Geometry: final body of the model. Coordinates: model frame, mm. Give positions to 0.01 mm unless a question says otherwise; leave off trailing zeros. Write each loop counter-clockwise with the first axis right and the second up, starting at its lowest first coordinate (ties: lowest second). Pieces come first, ordered by that corner, then holes.
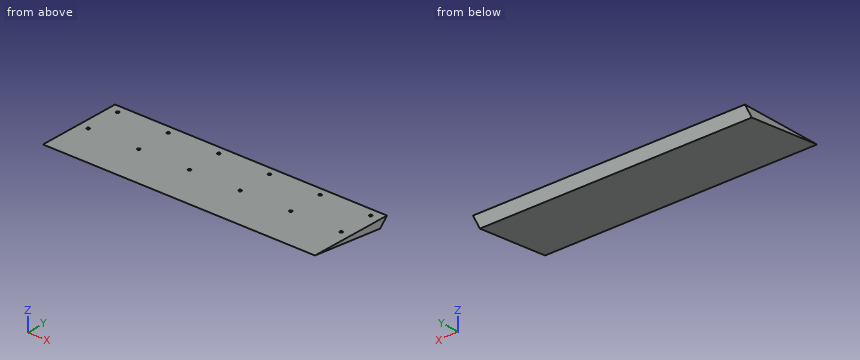
Autodesk Fusion 360 part; units mm, degrees
sketch "Sketch1" plane through (0, 0, 0) normal (0, 0, 1) x (1, 0, 0)
  line L0 (-217, 72) -> (217, 72)
  line L1 (217, 72) -> (217, -62)
  line L2 (217, -62) -> (-217, -62)
  line L3 (-217, -62) -> (-217, 72)
extrude "Extrude4" add sketch "Sketch1" against normal blind 230
sketch "Sketch4" plane through (-217, 0, 0) normal (-1, 0, 0) x (0, -1, 0)
  line L0 (62, 0) -> (-72, 0)
  line L1 (-72, 0) -> (-72, -230)
  line L2 (-72, -230) -> (62, -230)
  line L3 (62, -230) -> (62, 0)
  line L4 (62, 0) -> (-29, 0) construction
  line L5 (-72, 0) -> (-59.2555, -12.7445)
  line L6 (-72, 0) -> (-53.9766, 0) construction
  line L7 (62, 0) -> (-59.2555, -12.7445)
  line L8 (62, 0) -> (-59.9234, 0) construction
  dimension "d30" = 45
  dimension "d31" = 6
extrude "Extrude5" cut sketch "Sketch4" against normal blind 520 contours L1 L2 L3 L5 L7
sketch "Sketch5" plane through (0, 0, 0) normal (0, 0, 1) x (-1, 0, 0)
  line L0 (217, 62) -> (-217, 62)
  line L1 (-217, 62) -> (-217, -72)
  line L2 (-217, -72) -> (217, -72)
  line L3 (217, -72) -> (217, 62)
  circle A0 centre (202, -59.25) radius 2.25
  circle A1 centre (121.2, -59.25) radius 2.25
  circle A2 centre (40.4, -59.25) radius 2.25
  circle A3 centre (-40.4, -59.25) radius 2.25
  circle A4 centre (-121.2, -59.25) radius 2.25
  circle A5 centre (-202, -59.25) radius 2.25
  circle A6 centre (202, -4.5) radius 2.25
  circle A7 centre (121.2, -4.5) radius 2.25
  circle A8 centre (40.4, -4.5) radius 2.25
  circle A9 centre (-40.4, -4.5) radius 2.25
  circle A10 centre (-121.2, -4.5) radius 2.25
  circle A11 centre (-202, -4.5) radius 2.25
  dimension "d34" = 4.5
  dimension "d35" = 12.75
  dimension "d36" = 15
  dimension "d39" = -404
  dimension "d40" = 0
  dimension "d41" = 4.5
  dimension "d42" = 66.5
  dimension "d43" = 15
  dimension "d46" = -404
  dimension "d47" = 0
extrude "Extrude6" cut sketch "Sketch5" against normal blind 6 contours A0 | A1 | A2 | A3 | A4 | A5 | A6 | A7 | A8 | A9 | A10 | A11
Q1. Section B-B on x = -103. Output: boundary loops of the cut face in (y, z), plus the area to 3 significant figures.
Filled sheet:
outline: (-62, 0) - (59.26, -12.74) - (72, 0) - close
area: 854 mm2
Q2. Section C-C on y = 24. Output: boundary loops of the cut face in (x, z).
Filled sheet:
outline: (-217, -9.04) - (217, -9.04) - (217, 0) - (-217, 0) - close
Q3. Section D-D on y = -38.5. Output: boundary loops of the cut face in (x, z).
Filled sheet:
outline: (-217, -2.47) - (217, -2.47) - (217, 0) - (-217, 0) - close
Q4. Ray query, line 1 along Z through (x, y) = (184, -47.5); line 2 along Z through (x, y) = (-14.5, -40.5). Return the intervals inside material, ascending.
Filled sheet:
line 1: z = -1.52 to 0
line 2: z = -2.26 to 0
Q5. Section A-A on z = -2. Count the separate pieces of the cut face and the enclosed holes in it, plus the area to 3 significant figures.
Filled sheet:
separate pieces: 1
enclosed holes: 12
area: 48,800 mm2
Q6. Pin query (flat end, axial travel): P1, Ø2.5, axis at x = 202, y = 59.25, coming from the +Z side; P2, Ø6, axis at x = 66.5, y = -16, coming from the -Z side; P3, Ø3.5, axis at x = 40.4, y = 4.5, coming from the -Z side. Return the tip coordinate at first contact, or that it passes through.
Filled sheet:
P1: stops at z = -6
P2: stops at z = -5.15
P3: stops at z = -7.17
